from build123d import *

# Parameters (mm, degrees)
F0_W     = 120
F0_H     = 80
F0_R     = 1.5
F1_DEPTH = 5


with BuildPart() as f1:
    # F0 (on Front) → F1 (new body)
    with BuildSketch(Plane.XZ):
        with Locations((-10, 0)):
            Rectangle(F0_W, F0_H)
        with Locations((29, -5)):
            Circle(F0_R, mode=Mode.SUBTRACT)
        with Locations((-37, 0)):
            Circle(F0_R, mode=Mode.SUBTRACT)
        with Locations((-49, 29)):
            Circle(F0_R, mode=Mode.SUBTRACT)
        with Locations((-32, 30)):
            Circle(F0_R, mode=Mode.SUBTRACT)
        with Locations((-16, 30)):
            Circle(F0_R, mode=Mode.SUBTRACT)
        Circle(F0_R, mode=Mode.SUBTRACT)
        with Locations((32, 0)):
            Circle(F0_R, mode=Mode.SUBTRACT)
        with Locations((29, 4)):
            Circle(F0_R, mode=Mode.SUBTRACT)
        with Locations((29, 13)):
            Circle(F0_R, mode=Mode.SUBTRACT)
        with Locations((10, 30)):
            Circle(F0_R, mode=Mode.SUBTRACT)
    extrude(amount=F1_DEPTH)


solid = f1.part
Could you check a few things on this model? Use its own coordinates, in mm. Give positions to 0.01 mm unless a question says otherwise; leave off trailing zeros. Order: outer loops, then holes, each group sorted by start corner. A loop starts at its lowest first (then second) coordinate and runs counter-clockwise, first axis right, second up.
1. Suppose I cut it at A-A (x = 29). List the corners of the cut face in (y, z) for me, plus the area to 3 significant figures.
2. Suppose I cut it at C-C (x = 0). List the corners of the cut face in (y, z) for me.
3. I need wall thicknesses on L1, parallel to Z at x = 29, y = -2.9; L2, parallel to Z at x = -32, y = -2.6; L3, parallel to Z at x = -49, y = -1.05. Which ranges of each line are inside material? Lowest first, please.
4. Suppose I cut it at B-B (z = 13). List the corners of the cut face in (x, y) for me, plus the area to 3 significant figures.
5. We'd pull the mould along Z, two halves only. Please class faces 1 (the cylindrical face through (27.5, -2.46, 4.07)), 2 (the flat face through (-11, -2, -40)), 3 (the flat face through (-11, 0, 1)): pulls with the +Z half, pulls with the -Z half, needs draft (parallel to the pull), parting line crosses it, or undercut.
Solved:
1. outline: (-5, -40) - (0, -40) - (0, -6.5) - (-5, -6.5) - close; (-5, -3.5) - (0, -3.5) - (0, 2.5) - (-5, 2.5) - close; (-5, 5.5) - (0, 5.5) - (0, 11.5) - (-5, 11.5) - close; (-5, 14.5) - (0, 14.5) - (0, 40) - (-5, 40) - close
1. area: 355 mm2
2. outline: (-5, -40) - (0, -40) - (0, -1.5) - (-5, -1.5) - close; (-5, 1.5) - (0, 1.5) - (0, 40) - (-5, 40) - close
3. L1: z = -40 to -6.5, -3.5 to 2.5, 5.5 to 11.5, 14.5 to 40
3. L2: z = -40 to 28.5, 31.5 to 40
3. L3: z = -40 to 27.5, 30.5 to 40
4. outline: (-70, -5) - (27.5, -5) - (27.5, 0) - (-70, 0) - close; (30.5, -5) - (50, -5) - (50, 0) - (30.5, 0) - close
4. area: 585 mm2
5. face 1: undercut
5. face 2: pulls with the -Z half
5. face 3: needs draft
